from build123d import *

# Parameters (mm, degrees)
F1_DEPTH = 25.4
F3_DEPTH = 34.036
F5_DEPTH = 11.938


with BuildPart() as f1:
    # F0 (on Top) → F1 (new body)
    with BuildSketch(Plane.XY):
        with BuildLine():
            Line((17.636783421, 0.8561543655), (-2.8872299848, 0.8561543655))
            ThreePointArc((-2.8872299848, 0.8561543655), (-25.1709409058, -21.4275565556), (-47.4546518269, 0.8561543655))
            Line((-47.4546518269, 0.8561543655), (-67.9786652327, 0.8561543655))
            Line((-67.9786652327, 0.8561543655), (-67.9786652327, -10.787546169))
            Line((-67.9786652327, -10.787546169), (-77.1236439758, -10.787546169))
            ThreePointArc((-77.1236439758, -10.787546169), (-25.1709409058, -52.3853625026), (26.7817621641, -10.787546169))
            Line((26.7817621641, -10.787546169), (17.636783421, -10.787546169))
            Line((17.636783421, -10.787546169), (17.636783421, 0.8561543655))
        make_face()
        with BuildLine():
            ThreePointArc((-47.4546518269, 0.8561543655), (-25.1709409058, 23.1398652865), (-2.8872299848, 0.8561543655))
            Line((-2.8872299848, 0.8561543655), (17.636783421, 0.8561543655))
            Line((17.636783421, 0.8561543655), (17.636783421, 12.4998548999))
            Line((17.636783421, 12.4998548999), (26.7817621641, 12.4998548999))
            ThreePointArc((26.7817621641, 12.4998548999), (-25.1709409058, 54.0976712335), (-77.1236439758, 12.4998548999))
            Line((-77.1236439758, 12.4998548999), (-67.9786652327, 12.4998548999))
            Line((-67.9786652327, 12.4998548999), (-67.9786652327, 0.8561543655))
            Line((-67.9786652327, 0.8561543655), (-47.4546518269, 0.8561543655))
        make_face()
        with BuildLine():
            Line((-67.9786652327, -10.787546169), (-67.9786652327, 0.8561543655))
            Line((-67.9786652327, 0.8561543655), (-78.4124577739, 0.8561543655))
            ThreePointArc((-78.4124577739, 0.8561543655), (-78.0892734346, -5.0012512706), (-77.1236439758, -10.787546169))
            Line((-77.1236439758, -10.787546169), (-67.9786652327, -10.787546169))
        make_face()
        with BuildLine():
            Line((-78.4124577739, 0.8561543655), (-67.9786652327, 0.8561543655))
            Line((-67.9786652327, 0.8561543655), (-67.9786652327, 12.4998548999))
            Line((-67.9786652327, 12.4998548999), (-77.1236439758, 12.4998548999))
            ThreePointArc((-77.1236439758, 12.4998548999), (-78.0892734346, 6.7135600016), (-78.4124577739, 0.8561543655))
        make_face()
        with BuildLine():
            Line((-82.7045142651, 0.8561543655), (-78.4124577739, 0.8561543655))
            ThreePointArc((-78.4124577739, 0.8561543655), (-78.0892734346, 6.7135600016), (-77.1236439758, 12.4998548999))
            Line((-77.1236439758, 12.4998548999), (-82.7045142651, 12.4998548999))
            Line((-82.7045142651, 12.4998548999), (-82.7045142651, 0.8561543655))
        make_face()
        with BuildLine():
            ThreePointArc((-77.1236439758, -10.787546169), (-78.0892734346, -5.0012512706), (-78.4124577739, 0.8561543655))
            Line((-78.4124577739, 0.8561543655), (-82.7045142651, 0.8561543655))
            Line((-82.7045142651, 0.8561543655), (-82.7045142651, -10.787546169))
            Line((-82.7045142651, -10.787546169), (-77.1236439758, -10.787546169))
        make_face()
        with BuildLine():
            ThreePointArc((26.7817621641, 12.4998548999), (27.747391623, 6.7135600016), (28.0705759622, 0.8561543655))
            Line((28.0705759622, 0.8561543655), (32.3626324534, 0.8561543655))
            Line((32.3626324534, 0.8561543655), (32.3626324534, 12.4998548999))
            Line((32.3626324534, 12.4998548999), (26.7817621641, 12.4998548999))
        make_face()
        with BuildLine():
            Line((32.3626324534, 0.8561543655), (28.0705759622, 0.8561543655))
            ThreePointArc((28.0705759622, 0.8561543655), (27.747391623, -5.0012512706), (26.7817621641, -10.787546169))
            Line((26.7817621641, -10.787546169), (32.3626324534, -10.787546169))
            Line((32.3626324534, -10.787546169), (32.3626324534, 0.8561543655))
        make_face()
        with BuildLine():
            Line((28.0705759622, 0.8561543655), (17.636783421, 0.8561543655))
            Line((17.636783421, 0.8561543655), (17.636783421, -10.787546169))
            Line((17.636783421, -10.787546169), (26.7817621641, -10.787546169))
            ThreePointArc((26.7817621641, -10.787546169), (27.747391623, -5.0012512706), (28.0705759622, 0.8561543655))
        make_face()
        with BuildLine():
            Line((17.636783421, 12.4998548999), (17.636783421, 0.8561543655))
            Line((17.636783421, 0.8561543655), (28.0705759622, 0.8561543655))
            ThreePointArc((28.0705759622, 0.8561543655), (27.747391623, 6.7135600016), (26.7817621641, 12.4998548999))
            Line((26.7817621641, 12.4998548999), (17.636783421, 12.4998548999))
        make_face()
    extrude(amount=F1_DEPTH)

    # F2 (on face) → F3 (join)
    with BuildSketch(Plane.XY.offset(25.4)):
        Polygon((-77.1236439758, 12.4998548999), (-82.7045142651, 12.4998548999), (-82.7045142651, -10.787546169), (-77.1236439758, -10.787546169), (-72.7896168828, -10.787546169), (-72.7896168828, 12.4998548999), align=None)
        Polygon((32.3626324534, 12.4998548999), (26.7817621641, 12.4998548999), (23.2018940151, 12.4998548999), (23.2018940151, -10.787546169), (26.7817621641, -10.787546169), (32.3626324534, -10.787546169), align=None)
    extrude(amount=F3_DEPTH)

    # F4 (on face) → F5 (join)
    with BuildSketch(Plane.XY.offset(59.436)):
        with BuildLine():
            Line((-46.8474674883, 0.8561543655), (-72.7896168828, 0.8561543655))
            Line((-72.7896168828, 0.8561543655), (-72.7896168828, -10.787546169))
            Line((-72.7896168828, -10.787546169), (-79.5839477761, -10.787546169))
            ThreePointArc((-79.5839477761, -10.787546169), (-18.9982000681, -54.5411442591), (31.1630347279, 0.8561543655))
            Line((31.1630347279, 0.8561543655), (-2.8639275667, 0.8561543655))
            ThreePointArc((-2.8639275667, 0.8561543655), (-9.4154283034, -14.4917875948), (-24.8556975275, -20.8226303985))
            ThreePointArc((-24.8556975275, -20.8226303985), (-40.2959667516, -14.4917875948), (-46.8474674883, 0.8561543655))
        make_face()
        with BuildLine():
            Line((-72.7896168828, 12.4998548999), (-72.7896168828, 0.8561543655))
            Line((-72.7896168828, 0.8561543655), (-46.8474674883, 0.8561543655))
            ThreePointArc((-46.8474674883, 0.8561543655), (-40.5188840302, 16.611668132), (-24.8556975275, 23.1654282143))
            ThreePointArc((-24.8556975275, 23.1654282143), (-9.3035702594, 16.7235261761), (-2.8616682211, 1.1713989079))
            ThreePointArc((-2.8616682211, 1.1713989079), (-2.8622330648, 1.0137725886), (-2.8639275667, 0.8561543655))
            Line((-2.8639275667, 0.8561543655), (31.1630347279, 0.8561543655))
            ThreePointArc((31.1630347279, 0.8561543655), (31.1636999848, 1.0137760127), (31.1639217377, 1.1713989079))
            ThreePointArc((31.1639217377, 1.1713989079), (-19.1619844457, 56.9009186794), (-79.717923398, 12.4998548999))
            Line((-79.717923398, 12.4998548999), (-72.7896168828, 12.4998548999))
        make_face()
    extrude(amount=-F5_DEPTH)


solid = f1.part
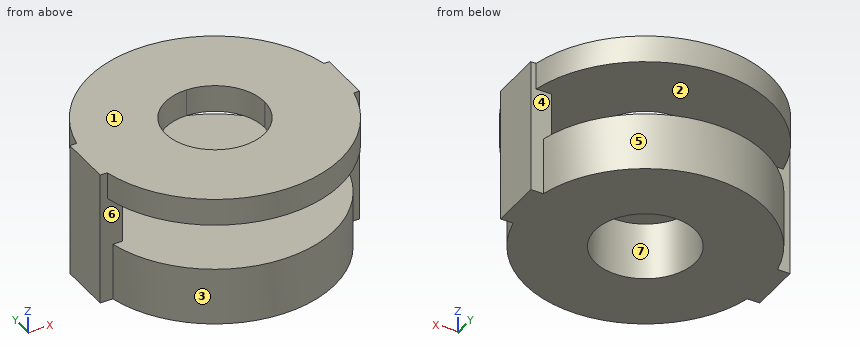
The listing builds one solid part. Answer for the finished solid, in the listing's coordinates (mm). Face numbers are marked on the shaded views. A direction names the side the tool comes from. Round coordinates to 2 decimals unless told otherwise and drop trailing zeros. Order: outer loops, then holes, each group sorted by start corner. A loop starts at its lowest first (then second) coordinate and runs counter-clockwise, first axis right, second up. Notation, with made-up numbers: (17.5, 24.25) -> (64.5, 24.25) arc R28 cw to (64.5, 42.25) -> close; hole circle Ø5 at (73, 16.25). An arc over 180 degrees is marked (long way). Put each result on its own line as item: value.
Q1. Which of the six approach directions +Z, -Z, +X, -X, +Y, -Y give full straight-line access (tool end or side, diameter ignored) to the marked faces 4, 5, 6 and 7?
Results list:
face 4: +X, +Y
face 5: -Z, +Y
face 6: -X, -Y
face 7: -Z
Q2. Section A-A, the plane z = 44 is taken. Write down the section's boundary in (x, y).
Results list:
outline: (-82.7, -10.79) -> (-72.79, -10.79) -> (-72.79, 12.5) -> (-82.7, 12.5) -> close; (23.2, -10.79) -> (32.36, -10.79) -> (32.36, 12.5) -> (23.2, 12.5) -> close
Q3. Section B-B, the plane x = -71 is taken. Write down the section's boundary in (y, z), and give its area (3 significant figures).
Results list:
outline: (-30.59, 47.5) -> (32.93, 47.5) -> (32.93, 59.44) -> (-30.59, 59.44) -> close; (-26.24, 0) -> (27.96, 0) -> (27.96, 25.4) -> (-26.24, 25.4) -> close
area: 2,140 mm^2
Q4. Section C-C, the plane x = -37 is taken. Write down the section's boundary in (y, z).
Results list:
outline: (-53.52, 47.5) -> (-17.17, 47.5) -> (-17.17, 59.44) -> (-53.52, 59.44) -> close; (-51.05, 0) -> (-18.03, 0) -> (-18.03, 25.4) -> (-51.05, 25.4) -> close; (19.51, 47.5) -> (55.86, 47.5) -> (55.86, 59.44) -> (19.51, 59.44) -> close; (19.74, 0) -> (52.77, 0) -> (52.77, 25.4) -> (19.74, 25.4) -> close
Q5. Determine the mould class of the marked faces 1, 2 and 3 for opening direction Z: pulls with the +Z half, pulls with the -Z half, needs draft (parallel to the pull), parting line crosses it, or undercut.
Results list:
face 1: pulls with the +Z half
face 2: undercut
face 3: needs draft
Q6. Consider line 1 along Z through (x, y) = (14, -34); line 2 along Y through (x, z) = (-25.5, 23); line 3 along X through (y, z) = (-18.5, 56). Determine where each line is inside the solid, lowest interval first.
Results list:
line 1: 0 to 25.4, 47.5 to 59.44
line 2: -52.38 to -21.43, 23.14 to 54.1
line 3: -77.31 to -34.69, -15.02 to 27.6
Q7. Section D-D, the plane z = 9.5 is taken. Write down the section's boundary in (x, y), and give its area (3 significant figures).
Results list:
outline: (-82.7, -10.79) -> (-77.12, -10.79) arc R53.24 ccw to (26.78, -10.79) -> (32.36, -10.79) -> (32.36, 12.5) -> (26.78, 12.5) arc R53.24 ccw to (-77.12, 12.5) -> (-82.7, 12.5) -> close; hole circle Ø44.57 at (-25.17, 0.86)
area: 7,570 mm^2
Q8. Each of these flat-tipped pins is pushed along its axis until it touches: P1, Ø4.5, axis at x = 29, z = 36, coming from the -Y side; P2, Ø6, axis at x = -71, z = 47.5, coming from the -Y side; P3, Ø5, axis at x = -76.5, z = 43.5, coming from the +Y side. Where does it stop, or does it pass through?
Results list:
P1: y = -10.79
P2: y = -34.56
P3: y = 12.5
